```python
from build123d import *

# Parameters (mm, degrees)
F1_DEPTH = 19.05
F2_W     = 19.05
F2_H     = 18.12971
F3_DEPTH = 38.1
F4_R     = 5.08
F5_SIZE  = 5.08
F6_R     = 12.7


with BuildPart() as f1:
    # F0 (on Front) → F1 (new body)
    with BuildSketch(Plane.XZ):
        Polygon((0, 38.1), (0, 0), (38.1, 0), (38.1, 38.1), (38.1, 57.15), (19.05, 57.15), (19.05, 38.1), align=None)
    extrude(amount=F1_DEPTH)

    # F2 (on face) → F3 (join)
    with BuildSketch(Plane.XZ.offset(19.05)):
        with Locations((28.575, 29.035145)):
            Rectangle(F2_W, F2_H)
    extrude(amount=F3_DEPTH)

    # F4
    f4_edges = [f1.edges().sort_by_distance(p)[0] for p in [
        (38.1, -38.1, 38.1),
    ]]
    fillet(f4_edges, radius=F4_R)

    # F5
    f5_edges = [f1.edges().sort_by_distance(p)[0] for p in [
        (26.035, -57.15, 38.1),
    ]]
    chamfer(f5_edges, length=F5_SIZE)

    # F6
    f6_edges = [f1.edges().sort_by_distance(p)[0] for p in [
        (38.1, -9.525, 57.15),
    ]]
    fillet(f6_edges, radius=F6_R)


solid = f1.part
```
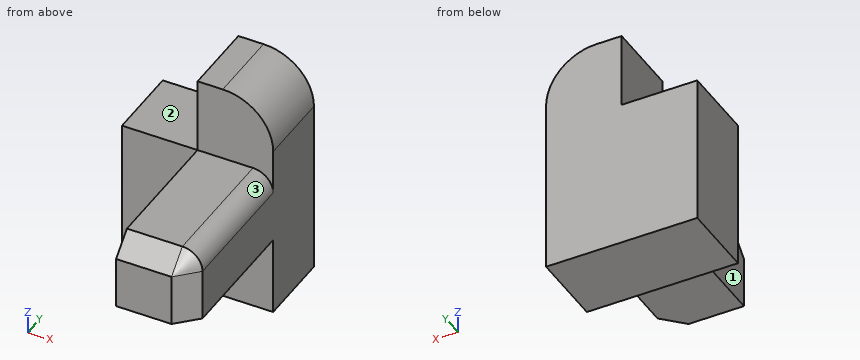
Design review of the part built by this model. Coordinates are the model's own, in mm. Face numbers are marked on the shaded views. A direction names the side the tool comes from. Round coordinates to 2 decimals unless told otherwise and drop trailing zeros. Write each loop counter-clockwise with the first axis right and the second up, starting at its lowest first coordinate (ties: lowest second). Pieces come first, ordered by that corner, then holes. Notation, with made-up numbers: (74, 21.5) -> (102, 21.5) arc R19 cw to (102, 42.5) -> close; hole circle Ø8 at (46, 4). An arc over 180 degrees is marked (long way). Answer in a Markdown table with one row per item.
Q1. To check wall thickness, follow L1, parallel to Z at x = 19.5, y = -45; L2, parallel to Y at x = 26.5, z = 46; L3, parallel to Z at x = 17, y = -3.5. State the ranges of each line that lie inside material, in increasing order. Write a range as [from, to].
The answers:
| item | result |
|---|---|
| L1 | [19.97, 38.1] |
| L2 | [-19.05, 0] |
| L3 | [0, 38.1] |
Q2. Clearance check with flat-ended pins moving along their axes: pin 1 Ø7 at (x, y) = (28.5, -29) entering from +Z; pin 2 Ø1 at (y, z) = (-28.5, 37) entering from -X; pin 3 Ø9.5 at (x, y) = (24, -43) entering from -Z; pin 4 Ø3 at (x, z) = (32, 44.5) entering from +Y. State where each tip first meets the part, or that it passes through.
The answers:
| item | result |
|---|---|
| pin 1 | z = 38.1 |
| pin 2 | x = 19.05 |
| pin 3 | z = 19.97 |
| pin 4 | y = 0 |
Q3. For the marked faces 1, 2 and 3, list the 3-axis set-ups (+Z, -Z, +X, -X, +Y, -Y) from which the entire face can be reached by the end or side of a thin tool; tool diameter is ignored.
The answers:
| item | result |
|---|---|
| face 1 | +Z, -Z, -X, -Y |
| face 2 | +Z, -X, +Y, -Y |
| face 3 | +Z, +X, -Y |
Q4. Take a section at D-D, the plane y = -45. State the section outline as (x, z) points, then the cut area to 3 significant figures.
The answers:
| item | result |
|---|---|
| outline | (19.05, 19.97) -> (38.1, 19.97) -> (38.1, 33.02) arc R5.08 ccw to (33.02, 38.1) -> (19.05, 38.1) -> close |
| area | 340 mm² |
Q5. Take a section at A-A, the plane z = 26. State the section outline as (x, y) points.
The answers:
| item | result |
|---|---|
| outline | (0, -19.05) -> (19.05, -19.05) -> (19.05, -57.15) -> (33.02, -57.15) -> (38.1, -52.07) -> (38.1, 0) -> (0, 0) -> close |
Q6. Take a section at C-C, the plane x = 27.5. State the section outline as (y, z) points, then the cut area to 3 significant figures.
The answers:
| item | result |
|---|---|
| outline | (-57.15, 19.97) -> (-19.05, 19.97) -> (-19.05, 0) -> (0, 0) -> (0, 56.98) -> (-19.05, 56.98) -> (-19.05, 38.1) -> (-52.07, 38.1) -> (-57.15, 33.02) -> close |
| area | 1,760 mm² |
Q7. Take a section at B-B, the plane y = -10. State the section outline as (x, z) points, then the cut area to 3 significant figures.
The answers:
| item | result |
|---|---|
| outline | (0, 0) -> (38.1, 0) -> (38.1, 44.45) arc R12.7 ccw to (25.4, 57.15) -> (19.05, 57.15) -> (19.05, 38.1) -> (0, 38.1) -> close |
| area | 1,780 mm² |
